from build123d import *

# Parameters (mm, degrees)
SKETCH006_W                        = 78.2
SKETCH006_H                        = 70.2
PAD004_DEPTH                       = 1
SKETCH011_R                        = 1.7
POCKET004_DEPTH                    = 211.184539
POCKET004_DEPTH_BACK               = 210.184539
SKETCH011_MIRRORED009_2_R          = 1.7
POCKET004_MIRRORED009_2_DEPTH      = 211.184539
POCKET004_MIRRORED009_2_DEPTH_BACK = -210.184539
SKETCH015_R                        = 1.7
PAD008_DEPTH                       = 22.3
SKETCH015_MIRRORED017_2_R          = 1.7
PAD008_MIRRORED017_2_DEPTH         = 22.3
SKETCH023_R                        = 3.5
POCKET014_DEPTH                    = 5
FILLET003_R                        = 5


with BuildPart() as part:
    # Sketch006 → Pad004 (new body)
    with BuildSketch(Plane.XY):
        Rectangle(SKETCH006_W, SKETCH006_H)
    extrude(amount=-PAD004_DEPTH)

    # Sketch011 → Pocket004 (cut, two sides)
    with BuildSketch(Plane.XY) as pocket004_sk:
        with Locations((-34.1, 30.1)):
            Circle(SKETCH011_R)
    pocket004 = extrude(amount=-POCKET004_DEPTH, mode=Mode.SUBTRACT) + extrude(pocket004_sk.sketch, amount=POCKET004_DEPTH_BACK, mode=Mode.SUBTRACT)

    # Sketch011 Mirrored009 2 → Pocket004 Mirrored009 2 (cut, two sides)
    with BuildSketch(Plane(origin=(0, 0, 0), x_dir=(-1, 0, 0), z_dir=(0, 0, -1))) as pocket004_mirrored009_2_sk:
        with Locations((-34.1, 30.1)):
            Circle(SKETCH011_MIRRORED009_2_R)
    pocket004_mirrored009_2 = extrude(amount=POCKET004_MIRRORED009_2_DEPTH, mode=Mode.SUBTRACT) + extrude(pocket004_mirrored009_2_sk.sketch, amount=-POCKET004_MIRRORED009_2_DEPTH_BACK, mode=Mode.SUBTRACT)

    # Mirrored010: Pocket004, Pocket004 Mirrored009 2 across Sketch011 H_Axis
    add(pocket004.mirror(Plane.ZX), mode=Mode.SUBTRACT)
    add(pocket004_mirrored009_2.mirror(Plane.ZX), mode=Mode.SUBTRACT)

    # Sketch015 → Pad008 (join)
    with BuildSketch(Plane.XY):
        with BuildLine():
            ThreePointArc((-34.1, 26.9), (-31.837258, 27.837258), (-30.9, 30.1))
            Line((-30.9, 30.1), (-30.9, 33.5))
            Line((-30.9, 33.5), (-37.5, 33.5))
            Line((-37.5, 33.5), (-37.5, 26.9))
            Line((-37.5, 26.9), (-34.1, 26.9))
        make_face()
        with Locations((-34.1, 30.1)):
            Circle(SKETCH015_R, mode=Mode.SUBTRACT)
    pad008 = extrude(amount=-PAD008_DEPTH)

    # Sketch015 Mirrored017 2 → Pad008 Mirrored017 2 (add)
    with BuildSketch(Plane(origin=(0, 0, 0), x_dir=(-1, 0, 0), z_dir=(0, 0, -1))):
        with BuildLine():
            ThreePointArc((-34.1, 26.9), (-31.837258, 27.837258), (-30.9, 30.1))
            Line((-30.9, 30.1), (-30.9, 33.5))
            Line((-30.9, 33.5), (-37.5, 33.5))
            Line((-37.5, 33.5), (-37.5, 26.9))
            Line((-37.5, 26.9), (-34.1, 26.9))
        make_face()
        with Locations((-34.1, 30.1)):
            Circle(SKETCH015_MIRRORED017_2_R, mode=Mode.SUBTRACT)
    pad008_mirrored017_2 = extrude(amount=PAD008_MIRRORED017_2_DEPTH)

    # Mirrored018: Pad008, Pad008 Mirrored017 2 across Sketch015 H_Axis
    add(pad008.mirror(Plane.ZX))
    add(pad008_mirrored017_2.mirror(Plane.ZX))

    # Sketch023 → Pocket014 (cut)
    with BuildSketch(Plane.XY):
        with Locations((-33, 0)):
            Circle(SKETCH023_R)
    extrude(amount=-POCKET014_DEPTH, mode=Mode.SUBTRACT)

    # Fillet003
    fillet003_edges = [part.edges().sort_by_distance(p)[0] for p in [
        (37.5, 33.5, -11.65),
        (39.1, 35.1, -0.5),
        (37.5, -33.5, -11.65),
        (39.1, -35.1, -0.5),
        (-39.1, -35.1, -0.5),
        (-37.5, -33.5, -11.65),
        (-37.5, 33.5, -11.65),
        (-39.1, 35.1, -0.5),
    ]]
    fillet(fillet003_edges, radius=FILLET003_R)


solid = part.part
Build history of the part. All positions in model axes, mm. A direction names the side the tool comes from. Round coordinates to 2 decimals unless told otherwise and drop trailing zeros. Order: outer loops, then holes, each group sorted by start corner. A loop starts at its lowest first (then second) coordinate and runs counter-clockwise, first axis right, second up. Notation, with made-up numbers: M 26.5,-15 L 69.5,-15 A26 cw 69.5,4 Z; hole C 55.5,45 d9. An arc over 180 degrees is marked long. Use CSV: the item, a comma, the result in double quotes. Start each with the question number.
(1) Drill centre lines: probe 1 along X at (y, z) = (-30.1, -15.75); probe 2 along Y at (x, z) = (-34.1, -15.5); probe 3 along Y at (x, z) = (-33, -15) (3 decimals). Where is each one in solid material? Low to high.
(2) Cut at C-C on x = -27. List the corners of the cut face in (y, z), then the cut area to 3 significant figures.
(3) Tool access for faces 5 (the face through (-36, -26.9, -12)), 6 (the face through (36, 32.07, -11.8)), 7 (the face through (-36, -32.07, -11.8)), 8 (the face through (30.9, -32, -12)): list every direction of +Z, -Z, +X, -X, +Y, -Y with a clear straight run to the whole face (end or side of a thin tool).
(4) Mould opens along Y. For faces 1 (the face through (-37.67, -33.6, -0.51)), 2 (the face through (31.862, -27.813, -11.501)), 3 (the face through (-37.67, 33.6, -0.51)), 4 (the face through (-1, 0, 0)) say: +Y half, -Y half, draft (parallel to the pull), parting line (faces both ways), or undercut.
(5) Cut at A-A on z = -20.75. List the corners of the cut face in (x, y), then the cut area to 3 significant figures.
(6) Flat gauge pins, fed straight in: P1, Ø0.8, axis at x = -31.5, z = -6.5, coming from the +Y side; P2, Ø5, axis at y = -22, z = -6.5, coming from the +X side; P3, Ø1.7, axis at x = 35, z = -15, coming from the -Y side; P4, Ø0.8, axis at y = -27.5, z = -9, coming from the +X side. Where does each tip first touch, or does it go through?
(7) Cut at B-B on y = -1.5. List the corners of the cut face in (x, z).
Findings:
1,probe 1,"x = -37.24 to -35.8, -32.4 to -30.9, 30.9 to 32.4, 35.8 to 37.24"
1,probe 2,"y = -33.24 to -31.8, -28.4 to -26.9, 26.9 to 28.4, 31.8 to 33.24"
1,probe 3,"y = -33.475 to -31.396, -28.804 to -27.095, 27.095 to 28.804, 31.396 to 33.475"
2,outline,"M -35.1,-1 L 35.1,-1 L 35.1,0 L -35.1,0 Z"
2,area,"70.2 mm^2"
3,face 5,"-Z, +X, -X"
3,face 6,"-Z, +X, +Y"
3,face 7,"-Z, -X, -Y"
3,face 8,"-Z, +Y, -Y"
4,face 1,"-Y half"
4,face 2,"undercut"
4,face 3,"+Y half"
4,face 4,"draft"
5,outline,"M -37.5,-28.5 A5 ccw -32.5,-33.5 L -30.9,-33.5 L -30.9,-30.1 A3.2 ccw -34.1,-26.9 L -37.5,-26.9 Z; M -37.5,26.9 L -34.1,26.9 A3.2 ccw -30.9,30.1 L -30.9,33.5 L -32.5,33.5 A5 ccw -37.5,28.5 Z; M 30.9,-33.5 L 32.5,-33.5 A5 ccw 37.5,-28.5 L 37.5,-26.9 L 34.1,-26.9 A3.2 ccw 30.9,-30.1 Z; M 30.9,30.1 A3.2 ccw 34.1,26.9 L 37.5,26.9 L 37.5,28.5 A5 ccw 32.5,33.5 L 30.9,33.5 Z; hole C -34.1,-30.1 d3.4; hole C -34.1,30.1 d3.4; hole C 34.1,-30.1 d3.4; hole C 34.1,30.1 d3.4"
5,area,"108 mm^2"
6,P1,"stops at y = 33.5"
6,P2,"passes through"
6,P3,"stops at y = -33.22"
6,P4,"stops at x = 37.5"
7,outline,"M -39.1,-1 L -36.16,-1 L -36.16,0 L -39.1,0 Z; M -29.84,-1 L 39.1,-1 L 39.1,0 L -29.84,0 Z"
